For this review, take the finished solid that the model builds, in its own axes (mm). Face numbers are marked on the shaded views. A direction names the side the tool comes from. Round coordinates to 2 decimals unless told otherwise and drop trailing zeros. Loops run counter-clockwise (first coordinate to the right, second up) from the corner with the lowest first, then second, coordinate; pieces in that order, holes last. Notation, with made-up numbers: (42, 5) -> (63, 5) arc R21 cw to (63, 21) -> close; hole circle Ø11 at (83.25, 79). An arc over 180 degrees is marked (long way). Write each question's results on one line, items separated by ' | '.
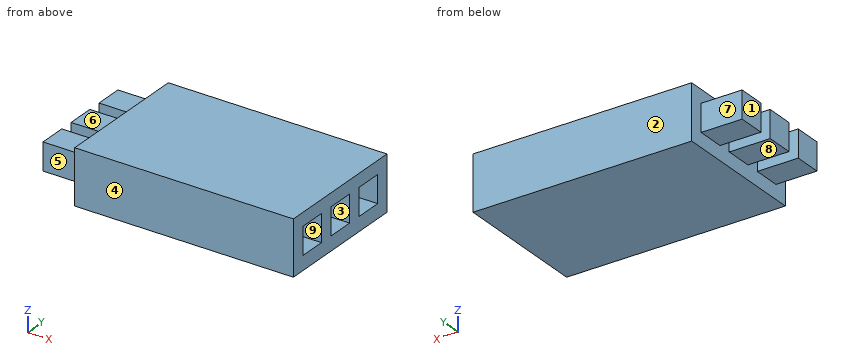
Autodesk Inventor part; units mm, degrees
ref_plane "YZ Plane" through (0, 0, 0) normal (1, 0, 0) x (0, 1, 0)
ref_plane "XZ Plane" through (0, 0, 0) normal (0, 1, 0) x (-1, 0, 0)
ref_plane "XY Plane" through (0, 0, 0) normal (0, 0, 1) x (1, 0, 0)
sketch "Sketch1" plane through (0, 0, 0) normal (1, 0, 0) x (0, 1, 0)
  line L0 (3.5, 1) -> (-1.5, 1)
  line L1 (-1.5, 1) -> (-1.5, -1)
  line L2 (-1.5, -1) -> (3.5, -1)
  line L3 (3.5, -1) -> (3.5, 1)
  point P0 (0, 0)
  dimension "d0" = 2
  dimension "d1" = 5
  dimension "d2" = 3.5
  dimension "d3" = 1
extrude "Extrusion1" add sketch "Sketch1" along normal blind 8
sketch "Sketch2" plane through (8, 0, 0) normal (1, 0, 0) x (0, 0, -1)
  line L0 (-0.5192, 3) -> (0.4808, 3)
  line L1 (0.4808, 3) -> (0.4808, 2)
  line L2 (0.4808, 2) -> (-0.5192, 2)
  line L3 (-0.5192, 2) -> (-0.5192, 3)
  line L4 (-0.5192, 1.5) -> (0.4808, 1.5)
  line L5 (0.4808, 1.5) -> (0.4808, 0.5)
  line L6 (0.4808, 0.5) -> (-0.5192, 0.5)
  line L7 (-0.5192, 0.5) -> (-0.5192, 1.5)
  line L8 (-0.5192, 0) -> (0.4808, 0)
  line L9 (0.4808, 0) -> (0.4808, -1)
  line L10 (0.4808, -1) -> (-0.5192, -1)
  line L11 (-0.5192, -1) -> (-0.5192, 0)
  line L12 (1, 3.5) -> (-1, 3.5)
  point P0 (0, 0)
  dimension "d6" = 1
  dimension "d7" = 1
  dimension "d8" = 1
  dimension "d9" = 1
  dimension "d10" = 1
  dimension "d11" = 0.5
  dimension "d12" = 0.5
  dimension "d13" = 0.5
extrude "Extrusion2" cut sketch "Sketch2" against normal blind 5
sketch "Sketch3" plane through (0, 0, 0) normal (-1, 0, 0) x (0, 0, 1)
  line L0 (-0.4808, 0) -> (-0.4808, -1)
  line L1 (0.5192, -1) -> (0.5192, 0)
  line L2 (-0.4808, -1) -> (0.5192, -1)
  line L3 (0.5192, -1) -> (0.5192, 0)
  line L4 (0.5192, 0) -> (-0.4808, 0)
  line L5 (-0.4808, 0) -> (-0.4808, -1)
  line L6 (-0.4808, 1.5) -> (-0.4808, 0.5)
  line L7 (0.5192, 1.5) -> (-0.4808, 1.5)
  line L8 (-0.4808, 0.5) -> (0.5192, 0.5)
  line L9 (0.5192, 0.5) -> (0.5192, 1.5)
  line L10 (0.5192, 1.5) -> (-0.4808, 1.5)
  line L11 (-0.4808, 1.5) -> (-0.4808, 0.5)
  line L12 (0.5192, 2) -> (0.5192, 3)
  line L13 (-0.4808, 1.9917) -> (0.5192, 1.9917)
  line L14 (0.5192, 1.9917) -> (0.5192, 3)
  line L15 (0.5192, 3) -> (-0.4808, 3)
  line L16 (-0.4808, 3) -> (-0.4808, 1.9917)
  point P0 (0, 0)
extrude "Extrusion3" add sketch "Sketch3" along normal blind 1.5
properties part number "konektorservomotora"
1. Consider section A-A (x = -0.75). State the section outline as (y, z) points.
Values found:
outline: (-1, -0.48) -> (0, -0.48) -> (0, 0.52) -> (-1, 0.52) -> close; (0.5, -0.48) -> (1.5, -0.48) -> (1.5, 0.52) -> (0.5, 0.52) -> close; (1.99, -0.48) -> (3, -0.48) -> (3, 0.52) -> (1.99, 0.52) -> close
2. Consider section D-D (z = -0.9). State the section outline as (x, y) points.
Values found:
outline: (0, -1.5) -> (8, -1.5) -> (8, 3.5) -> (0, 3.5) -> close
3. To check wall thickness, follow probe 1 along Y at (x, z) = (5.5, 0.3); probe 2 along Z at (x, y) = (6, 1.2); probe 3 along X at (y, z) = (1.3, 0.9). State the ranges of each line that lie inside material, in increasing order.
Values found:
probe 1: y = -1.5 to -1, 0 to 0.5, 1.5 to 2, 3 to 3.5 | probe 2: z = -1 to -0.48, 0.52 to 1 | probe 3: x = 0 to 8
4. For pin 1 (0.5 mm diameter, centred on x = -1, y = 1, fed in from +Z); pin 2 (0.5 mm diameter, centred on x = -0.5, z = 0, fed in from -Y); pin 3 (0.5 mm diameter, centred on y = -0.5, z = 0, fed in from +X), all flat-tipped, find the tip position at first contact; note any pin that passes through.
Values found:
pin 1: stops at z = 0.52 | pin 2: stops at y = -1 | pin 3: stops at x = 3
5. Consider section C-C (y = -0.75). State the section outline as (x, z) points, plus the area to 3 significant figures.
Values found:
outline: (-1.5, -0.48) -> (0, -0.48) -> (0, -1) -> (8, -1) -> (8, -0.48) -> (3, -0.48) -> (3, 0.52) -> (8, 0.52) -> (8, 1) -> (0, 1) -> (0, 0.52) -> (-1.5, 0.52) -> close | area: 12.5 mm2
6. Consider section B-B (x = 7.25). State the section outline as (y, z) points, plus the area to 3 significant figures.
Values found:
outline: (-1.5, -1) -> (3.5, -1) -> (3.5, 1) -> (-1.5, 1) -> close; hole (-1, -0.48) -> (0, -0.48) -> (0, 0.52) -> (-1, 0.52) -> close; hole (0.5, -0.48) -> (1.5, -0.48) -> (1.5, 0.52) -> (0.5, 0.52) -> close; hole (2, -0.48) -> (3, -0.48) -> (3, 0.52) -> (2, 0.52) -> close | area: 7.00 mm2
7. Draft analysis for pull direction Y (two halves, no side actions). For the marked faces 1, 2, 3 and 4, state which applies: released by +Y, released by -Y, zero draft, split by the parting line, or undercut.
Values found:
face 1: zero draft | face 2: released by +Y | face 3: undercut | face 4: released by -Y
8. Tool access review of the marked faces 5, 6, 7, 8 and 9: name each direction out of +Z, -Z, +X, -X, +Y, -Y from which nothing blocks a thin tool from reaching the whole face with its end or side.
Values found:
face 5: +Z, -Z, -X, -Y | face 6: +Z, -X, +Y, -Y | face 7: +Z, -Z, -X, +Y | face 8: -Z, -X, +Y, -Y | face 9: +X
